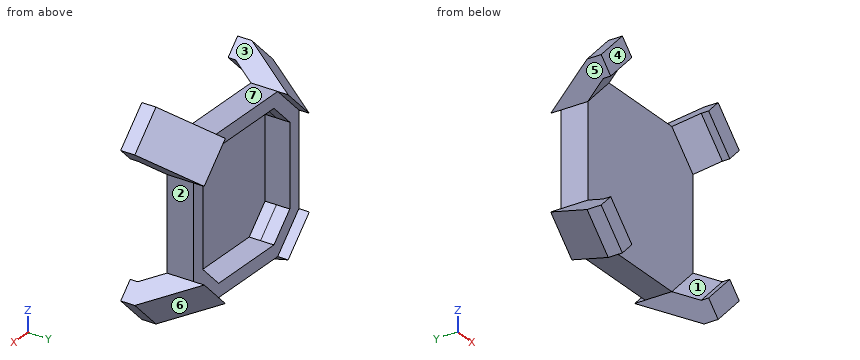
```python
from build123d import *

# Parameters (mm, degrees)
BOSS_EXTRUDE1_DEPTH      = 20
SHELL1_T                 = -10
SHELL1_THICKNESS_2_DEPTH = 8.5
BOSS_EXTRUDE2_DEPTH      = 33
MIRROR2_COPY_1_DEPTH     = 33


with BuildPart() as part:
    # Sketch1 → Boss-Extrude1 (new body)
    with BuildSketch(Plane(origin=(0, 0, 0), x_dir=(1, 0, 0), z_dir=(0, 1, 0))):
        Polygon((24.894532576, 77.33756703), (48.229056355, 54.003043251), (48.229056355, -15.232403626), (24.894532576, -38.566927405), (-44.340914301, -38.566927405), (-67.675438081, -15.232403626), (-67.675438081, 54.003043251), (-44.340914301, 77.33756703), align=None)
    extrude(amount=BOSS_EXTRUDE1_DEPTH)

    # Shell1
    shell1_openings = [part.faces().sort_by_distance(p)[0] for p in [
        (-9.723190863, 20, -19.385319812),
    ]]
    offset(amount=SHELL1_T, openings=shell1_openings, kind=Kind.INTERSECTION)

    # Shell1 thickness 2 face (on inner face of the shell) → Shell1 thickness 2 (cut)
    with BuildSketch(Plane(origin=(-9.723190863, 10, -19.385319812), x_dir=(0, 0, -1), z_dir=(0, -1, 0))):
        Polygon((30.475587815, 47.952247218), (47.952247218, 30.475587815), (47.952247218, -30.475587815), (30.475587815, -47.952247218), (-30.475587814, -47.952247218), (-47.952247217, -30.475587815), (-47.952247217, 30.475587815), (-30.475587814, 47.952247218), align=None)
    extrude(amount=SHELL1_THICKNESS_2_DEPTH, mode=Mode.SUBTRACT)

    # Sketch3 → Boss-Extrude2 (add)
    with BuildSketch(Plane(origin=(-6.836197415, 0, 6.836197415), x_dir=(0, -1, 0), z_dir=(0.7071067811865477, 0, -0.7071067811865475))):
        Polygon((-27.824686591, 86.039679274), (11.738008985, 111.769453035), (22.303053884, 111.769453035), (22.303053884, 96.927374932), (16.741172808, 96.927374932), (0, 86.039679274), align=None)
    boss_extrude2 = extrude(amount=BOSS_EXTRUDE2_DEPTH)

    # Mirror1: Boss-Extrude2 across plane
    add(boss_extrude2.mirror(Plane.XY.offset(-19.385319812)))

    # Mirror2: Boss-Extrude2 across plane
    add(boss_extrude2.mirror(Plane.ZY.offset(9.723190863)))

    # Mirror2 copy 1 sketch → Mirror2 copy 1 (add)
    with BuildSketch(Plane(origin=(-12.610184311, 0, -45.60683704), x_dir=(0, -1, 0), z_dir=(-0.7071067811865477, 0, 0.7071067811865475))):
        Polygon((-27.824686591, 86.039679274), (11.738008985, 111.769453035), (22.303053884, 111.769453035), (22.303053884, 96.927374932), (16.741172808, 96.927374932), (0, 86.039679274), align=None)
    extrude(amount=MIRROR2_COPY_1_DEPTH)


solid = part.part
```
The listing builds one solid part. Answer for the finished solid, in the listing's coordinates (mm). Face numbers are marked on the shaded views. A direction names the side the tool comes from. Give positions to 0.01 mm unless a question says otherwise; leave off trailing zeros. Order: outer loops, then holes, each group sorted by start corner. A loop starts at its lowest first (then second) coordinate and runs counter-clockwise, first axis right, second up. Notation, with made-up numbers: (71, 52) -> (122, 52) arc R4 ccw to (122, 59) -> close; hole circle Ø10 at (55, 50). An arc over 180 degrees is marked (long way). Answer as CSV lines item,"result". Start each with the question number.
Q1. Given pin 1 (9 mm diameter, centred on x = -11.5, y = 15.5, fed in from -Z); pin 2 (10 mm diameter, centred on y = 22, z = 27, fed in from -X); pin 3 (5.5 mm diameter, centred on y = 6.5, z = -32, fed in from -X), each flat-ended and moving along its own axis, determine where each tip first touches the part or whether it passes through.
Q2. Find the intervals of material crossed by L1, parallel to X at y = 16, z = -25; L2, parallel to Z at x = -33.5, y = 3; L3, parallel to Z at x = -12.5, y = 0.5, in increasing order.
Q3. Which of the six approach directions +Z, -Z, +X, -X, +Y, -Y give full straight-line access (tool end or side, diameter ignored) to the marked faces 1, 2 and 3?
Q4. A cutting plane is placed at A-A (y = 22.5). Determine the outline of the cut face in (x, z), then the cut area to 3 significant figures.
Q5. A cutting plane is placed at C-C (z = 2). Determine the outline of the cut face in (x, y), then the cut area to 3 significant figures.
Q6. A cutting plane is placed at B-B (y = 12). Determine the outline of the cut face in (x, z), then the cut area to 3 significant figures.
Q7. Determine the mould class of the marked faces 4, 5, 6 and 7 for opening direction X: pulls with the +X half, pulls with the -X half, needs draft (parallel to the pull), parting line crosses it, or undercut.
Q8. A cutting plane is placed at D-D (x = -9). Determine the outline of the cut face in (y, z), then the cut area to 3 significant figures.
Results found:
1,pin 1,"z = -77.34"
1,pin 2,"x = -68.06"
1,pin 3,"x = -67.68"
2,L1,"-67.68 to -57.68, 38.23 to 48.23"
2,L2,"-77.34 to -67.34, 28.57 to 38.57"
2,L3,"-77.34 to 38.57"
3,face 1,"-Y"
3,face 2,"+X, +Y, -Y"
3,face 3,"+Z, +Y, -Y"
4,outline,"(-70.12, -56.45) -> (-46.79, -79.79) -> (-44.34, -77.34) -> (-67.68, -54) -> close; (-70.12, 17.68) -> (-67.68, 15.23) -> (-44.34, 38.57) -> (-46.79, 41.02) -> close; (24.89, -77.34) -> (27.34, -79.79) -> (50.68, -56.45) -> (48.23, -54) -> close; (24.89, 38.57) -> (48.23, 15.23) -> (50.68, 17.68) -> (27.34, 41.02) -> close"
4,area,"457 mm2"
5,outline,"(-67.68, 0) -> (48.23, 0) -> (48.23, 20) -> (38.23, 20) -> (38.23, 1.5) -> (-57.68, 1.5) -> (-57.68, 20) -> (-67.68, 20) -> close"
5,area,"544 mm2"
6,outline,"(-74.95, -61.28) -> (-51.62, -84.61) -> (-44.34, -77.34) -> (24.89, -77.34) -> (32.17, -84.61) -> (55.51, -61.28) -> (48.23, -54) -> (48.23, 15.23) -> (55.51, 22.51) -> (32.17, 45.84) -> (24.89, 38.57) -> (-44.34, 38.57) -> (-51.62, 45.84) -> (-74.95, 22.51) -> (-67.68, 15.23) -> (-67.68, -54) -> close; hole (-57.68, -49.86) -> (-40.2, -67.34) -> (20.75, -67.34) -> (38.23, -49.86) -> (38.23, 11.09) -> (20.75, 28.57) -> (-40.2, 28.57) -> (-57.68, 11.09) -> close"
6,area,"5,120 mm2"
7,face 4,"needs draft"
7,face 5,"pulls with the -X half"
7,face 6,"pulls with the +X half"
7,face 7,"undercut"
8,outline,"(0, -77.34) -> (20, -77.34) -> (20, -67.34) -> (1.5, -67.34) -> (1.5, 28.57) -> (20, 28.57) -> (20, 38.57) -> (0, 38.57) -> close"
8,area,"544 mm2"
